Can you work these out from the model? Positions are in its coordinate system, mm. Face numbers are marked on the shaded views. A direction names the side the tool comes from. Coordinates: 2 decimals unless noted, no trailing zeros. Write each loop counter-clockwise with the first axis right and the second up, starting at its lowest first coordinate (ties: lowest second). Pieces come first, ordered by that corner, then holes.
```python
from build123d import *

# Parameters (mm, degrees)
BASE_FLANGE1_DEPTH           = 1
EDGE_FLANGE1_STRIP_W         = 7.2
EDGE_FLANGE1_STRIP_H         = 1
EDGE_FLANGE1_STRIP_CUT_DEPTH = 40
EDGE_FLANGE1_DEPTH           = 40
EDGE_FLANGE2_STRIP_W         = 7.2
EDGE_FLANGE2_STRIP_H         = 1
EDGE_FLANGE2_STRIP_CUT_DEPTH = 40
EDGE_FLANGE2_DEPTH           = 40
EDGE_FLANGE3_STRIP_W         = 7.2
EDGE_FLANGE3_STRIP_H         = 1
EDGE_FLANGE3_STRIP_CUT_DEPTH = 20
EDGE_FLANGE3_DEPTH           = 20
EDGE_FLANGE4_STRIP_W         = 7.2
EDGE_FLANGE4_STRIP_H         = 1
EDGE_FLANGE4_STRIP_CUT_DEPTH = 20
EDGE_FLANGE4_DEPTH           = 20
SKETCH18_R                   = 2.1
CUT_EXTRUDE1_DEPTH           = 6
SKETCH19_R                   = 2.1
CUT_EXTRUDE2_DEPTH           = 6
SKETCH20_R                   = 2.1
CUT_EXTRUDE3_DEPTH           = 50
SKETCH21_R                   = 2.25
CUT_EXTRUDE4_DEPTH           = 50


# Sheet-metal steps are written as plain solids
with BuildPart() as part:
    # Sketch1 → Base-Flange1 (new body)
    with BuildSketch(Plane.XY):
        Polygon((0, 0), (0, 3), (-40, 3), (-40, 0), (-20, 0), (-20, -37), (-18.16511543, -37), (0, -37), align=None)
    extrude(amount=-BASE_FLANGE1_DEPTH)

    # Edge-Flange1 strip (across the edge) → Edge-Flange1 strip cut (cut)
    with BuildSketch(Plane(origin=(0, 3, 0), x_dir=(0, -1, 0), z_dir=(-1, 0, 0))):
        with Locations((-1, -0.5)):
            Rectangle(EDGE_FLANGE1_STRIP_W, EDGE_FLANGE1_STRIP_H)
    extrude(amount=EDGE_FLANGE1_STRIP_CUT_DEPTH, mode=Mode.SUBTRACT)

    # Edge-Flange1 section (across the edge) → Edge-Flange1 (add)
    with BuildSketch(Plane(origin=(0, 3, 0), x_dir=(0, -1, 0), z_dir=(-1, 0, 0))):
        with BuildLine():
            Line((0, 1.6), (0, 67))
            Line((0, 67), (1, 67))
            Line((1, 67), (1, 1.6))
            ThreePointArc((1, 1.6), (1.46862915, 0.46862915), (2.6, 0))
            Line((2.6, 0), (2.6, -1))
            ThreePointArc((2.6, -1), (0.761522369, -0.238477631), (0, 1.6))
        make_face()
    extrude(amount=EDGE_FLANGE1_DEPTH)

    # Edge-Flange2 strip (across the edge) → Edge-Flange2 strip cut (cut)
    with BuildSketch(Plane(origin=(-40, 3, 67), x_dir=(0, 0, -1), z_dir=(1, 0, 0))):
        with Locations((-1, -0.5)):
            Rectangle(EDGE_FLANGE2_STRIP_W, EDGE_FLANGE2_STRIP_H)
    extrude(amount=EDGE_FLANGE2_STRIP_CUT_DEPTH, mode=Mode.SUBTRACT)

    # Edge-Flange2 section (across the edge) → Edge-Flange2 (add)
    with BuildSketch(Plane(origin=(-40, 3, 67), x_dir=(0, 0, -1), z_dir=(1, 0, 0))):
        with BuildLine():
            Line((0, 1.6), (0, 13))
            Line((0, 13), (1, 13))
            Line((1, 13), (1, 1.6))
            ThreePointArc((1, 1.6), (1.46862915, 0.46862915), (2.6, 0))
            Line((2.6, 0), (2.6, -1))
            ThreePointArc((2.6, -1), (0.761522369, -0.238477631), (0, 1.6))
        make_face()
    extrude(amount=EDGE_FLANGE2_DEPTH)

    # Edge-Flange3 strip (across the edge) → Edge-Flange3 strip cut (cut)
    with BuildSketch(Plane(origin=(-20, -37, 0), x_dir=(0, 1, 0), z_dir=(1, 0, 0))):
        with Locations((-1, -0.5)):
            Rectangle(EDGE_FLANGE3_STRIP_W, EDGE_FLANGE3_STRIP_H)
    extrude(amount=EDGE_FLANGE3_STRIP_CUT_DEPTH, mode=Mode.SUBTRACT)

    # Edge-Flange3 section (across the edge) → Edge-Flange3 (add)
    with BuildSketch(Plane(origin=(-20, -37, 0), x_dir=(0, 1, 0), z_dir=(1, 0, 0))):
        with BuildLine():
            Line((0, 1.6), (0, 24))
            Line((0, 24), (1, 24))
            Line((1, 24), (1, 1.6))
            ThreePointArc((1, 1.6), (1.46862915, 0.46862915), (2.6, 0))
            Line((2.6, 0), (2.6, -1))
            ThreePointArc((2.6, -1), (0.761522369, -0.238477631), (0, 1.6))
        make_face()
    extrude(amount=EDGE_FLANGE3_DEPTH)

    # Edge-Flange4 strip (across the edge) → Edge-Flange4 strip cut (cut)
    with BuildSketch(Plane(origin=(0, -37, 24), x_dir=(0, 0, -1), z_dir=(-1, 0, 0))):
        with Locations((-1, -0.5)):
            Rectangle(EDGE_FLANGE4_STRIP_W, EDGE_FLANGE4_STRIP_H)
    extrude(amount=EDGE_FLANGE4_STRIP_CUT_DEPTH, mode=Mode.SUBTRACT)

    # Edge-Flange4 section (across the edge) → Edge-Flange4 (add)
    with BuildSketch(Plane(origin=(0, -37, 24), x_dir=(0, 0, -1), z_dir=(-1, 0, 0))):
        with BuildLine():
            Line((0, 1.6), (0, 14))
            Line((0, 14), (1, 14))
            Line((1, 14), (1, 1.6))
            ThreePointArc((1, 1.6), (1.46862915, 0.46862915), (2.6, 0))
            Line((2.6, 0), (2.6, -1))
            ThreePointArc((2.6, -1), (0.761522369, -0.238477631), (0, 1.6))
        make_face()
    extrude(amount=EDGE_FLANGE4_DEPTH)

    # Sketch18 → Cut-Extrude1 (cut)
    with BuildSketch(Plane(origin=(0, 0, 66), x_dir=(-1, 0, 0), z_dir=(0, 0, -1))):
        with Locations((9, 10.3)):
            Circle(SKETCH18_R)
        with Locations((31, 10.3)):
            Circle(SKETCH18_R)
    extrude(amount=-CUT_EXTRUDE1_DEPTH, mode=Mode.SUBTRACT)

    # Sketch19 → Cut-Extrude2 (cut)
    with BuildSketch(Plane(origin=(0, 0, 23), x_dir=(-1, 0, 0), z_dir=(0, 0, -1))):
        with Locations((9.178318955, -41.637901039)):
            Circle(SKETCH19_R)
    extrude(amount=-CUT_EXTRUDE2_DEPTH, mode=Mode.SUBTRACT)

    # Sketch20 → Cut-Extrude3 (cut)
    with BuildSketch(Plane(origin=(0, 3, 0), x_dir=(1, 0, 0), z_dir=(0, 1, 0))):
        with Locations(Location((-9.153318955, -41.090231637, 0), (0, 0, 270))):
            Circle(SKETCH20_R)
        with Locations(Location((-9.153318955, -16.090231637, 0), (0, 0, 270))):
            Circle(SKETCH20_R)
    extrude(amount=-CUT_EXTRUDE3_DEPTH, mode=Mode.SUBTRACT)

    # Sketch21 → Cut-Extrude4 (cut)
    with BuildSketch(Plane.XZ.offset(-2)):
        with Locations(Location((-21.883318955, 41.090231637, 0), (0, 0, 270))):
            Circle(SKETCH21_R)
        with Locations(Location((-34.563318955, 41.090231637, 0), (0, 0, 270))):
            Circle(SKETCH21_R)
    extrude(amount=-CUT_EXTRUDE4_DEPTH, mode=Mode.SUBTRACT)


solid = part.part
```
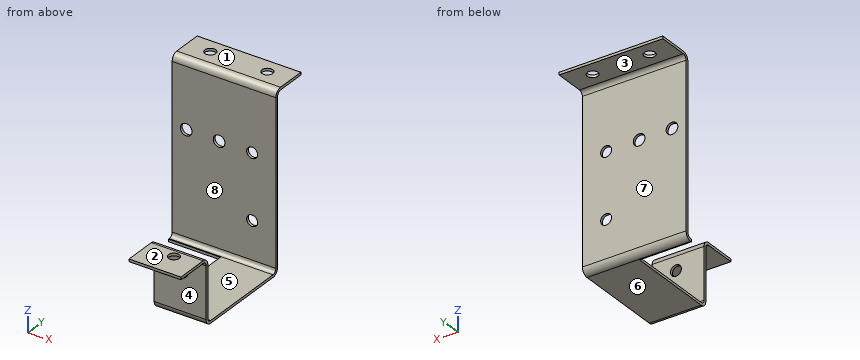
1. If we section it at C-C, the plane x = -31: List the corners of the cut face in (y, z) for me.
2. We'd pull the mould along Y, two halves only. Please class the marked faces 6, 7 and 8: released by +Y, released by -Y, zero draft, split by the parting line, or undercut.
3. If we section it at B-B, the plane y = 10.3: List the corners of the cut face in (x, z) for me.
4. Which directions (+Z, -Z, +X, -X, +Y, -Y) give clear straight access to the entire face, cutting with the end or side of a thin tool? Please do the marked faces 1, 2, 3, 4 and 5.
5. If we section it at D-D, the plane x = -17.5: List the corners of the cut face in (y, z) for me.
6. I'm going to push flat-ended pins straight in: P1, Ø6.5, axis at x = -9.15, z = 16.09, coming from the -Y side; P2, Ø12, axis at x = -16, y = 3.5, coming from the +Z side; P3, Ø0.8, axis at x = -30.5, z = -0.5, coming from the -Y side; P4, Ø4, axis at x = -29.5, z = 58, coming from the -Y side. Where does each tip first touch, or does it pass through?
7. If we section it at A-A, the plane z = 9.5: List the corners of the cut face in (x, y) for me, plus the area to 3 significant figures.
8. If I drill on L1, parallel to Y at x = -2, z = 18.5; L2, parallel to Y at x = -16, z = 47; L3, parallel to Z at x = -16.5, y = -16, over which ranges is the centre line in solid material (lowest first)?
Answers:
1. outline: (0, -1) - (0.4, -1) arc R2.6 ccw to (3, 1.6) - (3, 64.4) arc R1.6 cw to (4.6, 66) - (8.2, 66) - (8.2, 67) - (4.6, 67) arc R2.6 ccw to (2, 64.4) - (2, 1.6) arc R1.6 cw to (0.4, 0) - (0, 0) - close; (12.4, 66) - (16, 66) - (16, 67) - (12.4, 67) - close
2. face 6: zero draft
2. face 7: released by +Y
2. face 8: undercut
3. outline: (-40, 66) - (-33.1, 66) - (-33.1, 67) - (-40, 67) - close; (-28.9, 66) - (-11.1, 66) - (-11.1, 67) - (-28.9, 67) - close; (-6.9, 66) - (0, 66) - (0, 67) - (-6.9, 67) - close
4. face 1: +Z, +X, -X, +Y, -Y
4. face 2: +Z, +X, -X, -Y
4. face 3: -Z, +X, -X, +Y
4. face 4: -Z, +X, -X, -Y
4. face 5: +Z, +X, -X
5. outline: (-51, 23) - (-38.6, 23) arc R1.6 cw to (-37, 21.4) - (-37, 1.6) arc R2.6 ccw to (-34.4, -1) - (0.4, -1) arc R2.6 ccw to (3, 1.6) - (3, 64.4) arc R1.6 cw to (4.6, 66) - (16, 66) - (16, 67) - (4.6, 67) arc R2.6 ccw to (2, 64.4) - (2, 1.6) arc R1.6 cw to (0.4, 0) - (-34.4, 0) arc R1.6 cw to (-36, 1.6) - (-36, 21.4) arc R2.6 ccw to (-38.6, 24) - (-51, 24) - close
6. P1: stops at y = -37
6. P2: stops at z = 67
6. P3: stops at y = 0
6. P4: stops at y = 2
7. outline: (-40, 2) - (0, 2) - (0, 3) - (-40, 3) - close; (-20, -37) - (0, -37) - (0, -36) - (-20, -36) - close
7. area: 60.0 mm2
8. L1: y = -37 to -36, 2 to 3
8. L2: y = 2 to 3
8. L3: z = -1 to 0
